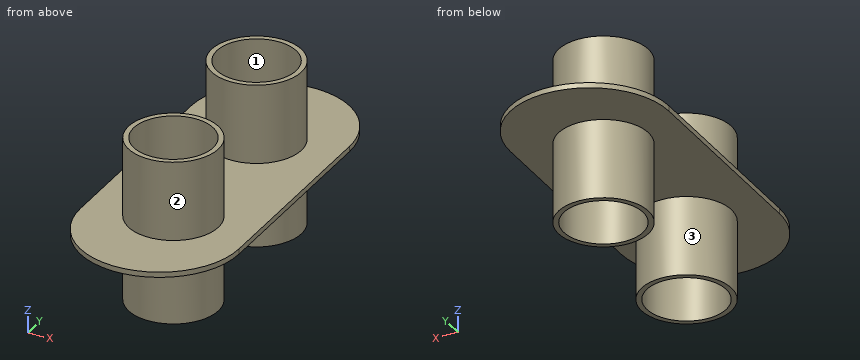
```python
from build123d import *

# Parameters (mm, degrees)
BOSS_EXTRUDE1_DEPTH     = 2.54
SKETCH5_R               = 21.59
BOSS_EXTRUDE5_DEPTH     = 38.1
BOSS_EXTRUDE6_START     = 38.1
SKETCH2_R               = 21.59
BOSS_EXTRUDE6_DEPTH     = 38.1
CUT_EXTRUDE2_DEPTH      = 125.718914363
CUT_EXTRUDE2_DEPTH_BACK = 125.718914363
SKETCH6_R               = 19.05


with BuildPart() as part:
    # Sketch1 → Boss-Extrude1 (new body)
    with BuildSketch(Plane.XY):
        with BuildLine():
            Line((38.1, 50.8), (0, 50.8))
            Line((0, 50.8), (-38.1, 50.8))
            ThreePointArc((-38.1, 50.8), (0, 12.7), (38.1, 50.8))
        make_face()
        with BuildLine():
            Line((-38.1, 50.8), (0, 50.8))
            Line((0, 50.8), (38.1, 50.8))
            ThreePointArc((38.1, 50.8), (0, 88.9), (-38.1, 50.8))
        make_face()
        with BuildLine():
            ThreePointArc((38.1, 50.8), (0, 12.7), (-38.1, 50.8))
            Line((-38.1, 50.8), (-38.1, -50.8))
            ThreePointArc((-38.1, -50.8), (0, -12.7), (38.1, -50.8))
            Line((38.1, -50.8), (38.1, 50.8))
        make_face()
        with BuildLine():
            ThreePointArc((38.1, -50.8), (0, -12.7), (-38.1, -50.8))
            Line((-38.1, -50.8), (0, -50.8))
            Line((0, -50.8), (38.1, -50.8))
        make_face()
        with BuildLine():
            Line((0, -50.8), (-38.1, -50.8))
            ThreePointArc((-38.1, -50.8), (0, -88.9), (38.1, -50.8))
            Line((38.1, -50.8), (0, -50.8))
        make_face()
    extrude(amount=BOSS_EXTRUDE1_DEPTH)

    # Sketch5 → Boss-Extrude5 (add)
    with BuildSketch(Plane(origin=(0, 0, 0), x_dir=(-1, 0, 0), z_dir=(0, 0, -1))):
        with Locations(Location((0, 38.1, 0), (0, 0, 180))):
            Circle(SKETCH5_R)
        with Locations(Location((0, -38.1, 0), (0, 0, 180))):
            Circle(SKETCH5_R)
    extrude(amount=BOSS_EXTRUDE5_DEPTH)

    # Sketch2 → Boss-Extrude6 (add)
    with BuildSketch(Plane.XY.offset(2.54).offset(BOSS_EXTRUDE6_START)):
        with Locations((0, 38.1)):
            Circle(SKETCH2_R)
        with Locations((0, -38.1)):
            Circle(SKETCH2_R)
    extrude(amount=-BOSS_EXTRUDE6_DEPTH)

    # Sketch6 → Cut-Extrude2 (cut, two sides: drawn at the far end of the back side and taken through both)
    with BuildSketch(Plane(origin=(0, 0, -38.1), x_dir=(-1, 0, 0), z_dir=(0, 0, -1)).offset(-CUT_EXTRUDE2_DEPTH_BACK)):
        with Locations((0, 38.1)):
            Circle(SKETCH6_R)
        with Locations((0, -38.1)):
            Circle(SKETCH6_R)
    extrude(amount=CUT_EXTRUDE2_DEPTH + CUT_EXTRUDE2_DEPTH_BACK, mode=Mode.SUBTRACT)


solid = part.part
```
For this review, take the finished solid that the model builds, in its own axes (mm). Face numbers are marked on the shaded views. A direction names the side the tool comes from. Coordinates: 2 decimals unless noted, no trailing zeros. Order: outer loops, then holes, each group sorted by start corner. A loop starts at its lowest first (then second) coordinate and runs counter-clockwise, first axis right, second up. Notation, with made-up numbers: (-14, 67.5) -> (30, 67.5) arc R23 ccw to (30, 92.5) -> close; hole circle Ø6 at (35, 26.25). An arc over 180 degrees is marked (long way). Answer as CSV lines item,"result".
Q1. We need section B-B (y = -38.1). State the section outline as (x, z) points, plus the area to 3 significant figures.
Model answer:
outline,"(-38.1, 0) -> (-21.59, 0) -> (-21.59, -38.1) -> (-19.05, -38.1) -> (-19.05, 40.64) -> (-21.59, 40.64) -> (-21.59, 2.54) -> (-38.1, 2.54) -> close; (19.05, -38.1) -> (21.59, -38.1) -> (21.59, 0) -> (38.1, 0) -> (38.1, 2.54) -> (21.59, 2.54) -> (21.59, 40.64) -> (19.05, 40.64) -> close"
area,"484 mm2"
Q2. We need section A-A (x = 0). State the section outline as (y, z) points, plus the area to 3 significant figures.
Model answer:
outline,"(-88.9, 0) -> (-59.69, 0) -> (-59.69, -38.1) -> (-57.15, -38.1) -> (-57.15, 40.64) -> (-59.69, 40.64) -> (-59.69, 2.54) -> (-88.9, 2.54) -> close; (-19.05, -38.1) -> (-16.51, -38.1) -> (-16.51, 0) -> (16.51, 0) -> (16.51, -38.1) -> (19.05, -38.1) -> (19.05, 40.64) -> (16.51, 40.64) -> (16.51, 2.54) -> (-16.51, 2.54) -> (-16.51, 40.64) -> (-19.05, 40.64) -> close; (57.15, -38.1) -> (59.69, -38.1) -> (59.69, 0) -> (88.9, 0) -> (88.9, 2.54) -> (59.69, 2.54) -> (59.69, 40.64) -> (57.15, 40.64) -> close"
area,"1,030 mm2"
Q3. Wall thickness on line 1 along Y through (x, z) = (0, 20); line 2 along Y through (x, z) = (9.5, -22); line 3 along Z through (x, y) = (25.5, -13.5): over which ranges is each line inside the solid? List them lowest first. Write a range as [from, to].
Model answer:
line 1,"y = [-59.69, -57.15], [-19.05, -16.51], [16.51, 19.05], [57.15, 59.69]"
line 2,"y = [-57.49, -54.61], [-21.59, -18.71], [18.71, 21.59], [54.61, 57.49]"
line 3,"z = [0, 2.54]"
Q4. We need section D-D (x = -14). State the section outline as (y, z) points.
Model answer:
outline,"(-86.23, 0) -> (-54.54, 0) -> (-54.54, -38.1) -> (-51.02, -38.1) -> (-51.02, 40.64) -> (-54.54, 40.64) -> (-54.54, 2.54) -> (-86.23, 2.54) -> close; (-25.18, -38.1) -> (-21.66, -38.1) -> (-21.66, 0) -> (21.66, 0) -> (21.66, -38.1) -> (25.18, -38.1) -> (25.18, 40.64) -> (21.66, 40.64) -> (21.66, 2.54) -> (-21.66, 2.54) -> (-21.66, 40.64) -> (-25.18, 40.64) -> close; (51.02, -38.1) -> (54.54, -38.1) -> (54.54, 0) -> (86.23, 0) -> (86.23, 2.54) -> (54.54, 2.54) -> (54.54, 40.64) -> (51.02, 40.64) -> close"
Q5. We need section C-C (z = -29). State the section outline as (x, y) points.
Model answer:
outline,"circle Ø43.18 at (0, -38.1); circle Ø43.18 at (0, 38.1); hole circle Ø38.1 at (0, -38.1); hole circle Ø38.1 at (0, 38.1)"
Q6. Clearance check with flat-ended pins moving along their axes: pin 1 Ø10 at (x, z) = (20.5, 5) entering from -Y; pin 2 Ø5 at (x, y) = (-14.5, 43) entering from +Z; pin 3 Ø3 at (x, y) = (-30.5, 37.5) entering from +Z; pin 4 Ø5 at (y, z) = (37, 12) entering from -X. State where each tip first meets the part, or that it passes through.
Model answer:
pin 1,"stops at y = -85.31"
pin 2,"passes through"
pin 3,"stops at z = 2.54"
pin 4,"stops at x = -21.59"
Q7. For the marked faces 1, 2 and 3, list the 3-axis set-ups (+Z, -Z, +X, -X, +Y, -Y) from which the entire face can be reached by the end or side of a thin tool; tool diameter is ignored.
Model answer:
face 1,"+Z, -Z"
face 2,"+Z"
face 3,"-Z"
